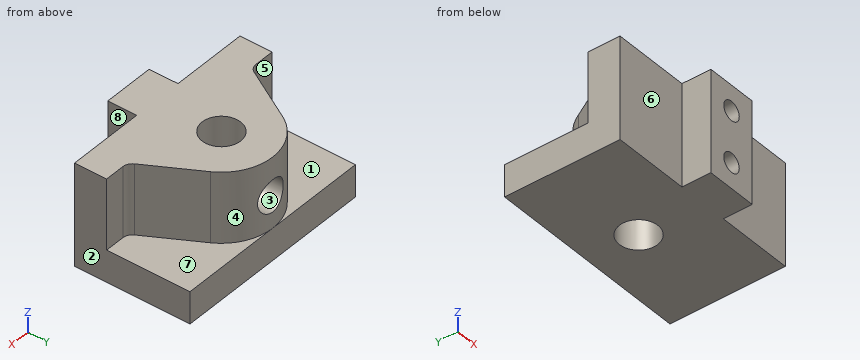
from build123d import *

# Parameters (mm, degrees)
BOSS_EXTRUDE1_DEPTH       = 36
CUT_EXTRUDE6_DEPTH        = 22
SKETCH11_R                = 6.000000000000001
CUT_EXTRUDE7_DEPTH        = 58.827329183593626
SKETCH12_W                = 16
SKETCH12_H                = 32
BOSS_EXTRUDE2_DEPTH       = 9
F_1_0MM_DOWEL_HOLE1_D     = 6
F_1_0MM_DOWEL_HOLE1_DEPTH = 16
F_1_0MM_DOWEL_HOLE1_TIP   = 1.8025818570826808


# Read off the part's stored shape, not the designer's step: CBORE for M6 Hex Socket Head Cap Screw2
with BuildPart() as part:
    # Sketch1 → Boss-Extrude1 (new body)
    with BuildSketch(Plane(origin=(0, 0, 0), x_dir=(1, 0, 0), z_dir=(0, 1, 0))):
        Polygon((-32.000000000000014, 16), (32, 16), (32, -16), (-32.00000000000001, -16), align=None)
    extrude(amount=BOSS_EXTRUDE1_DEPTH)

    # Sketch2 → Cut-Extrude6 (cut)
    with BuildSketch(Plane.XY.offset(16)):
        with BuildLine():
            Line((0.00047501965244123, 36), (-32.00000000000001, 36))
            Line((-32.00000000000001, 36), (-32.00000000000001, 10))
            Line((-32.00000000000001, 10), (-25.751640415984067, 10))
            ThreePointArc((-25.751640415984067, 10), (-24.238970505556754, 10.409280072626942), (-23.139037695662964, 11.5254468386081))
            Line((-23.139037695662964, 11.5254468386081), (-14.249494850462119, 27.275875122834456))
            ThreePointArc((-14.249494850462119, 27.275875122834453), (-8.35374541517065, 33.645768615897694), (0.00047501965243812, 36.00000000705136))
        make_face()
        with BuildLine():
            Line((31.999999999999993, 36), (0.00047501965244123, 36))
            ThreePointArc((0.00047501965243812, 36.00000000705136), (8.07302482579058, 33.814265808302636), (13.940018609128462, 27.85424246049306))
            Line((13.940018609128462, 27.85424246049306), (23.139425445581196, 11.527329539979691))
            ThreePointArc((23.139425445581196, 11.527329539979691), (24.239486779956046, 10.409825162265975), (25.753089868605628, 10))
            Line((25.753089868605628, 10), (32, 10.000000000000002))
            Line((32, 10.000000000000002), (32, 36))
        make_face()
    extrude(amount=-CUT_EXTRUDE6_DEPTH, mode=Mode.SUBTRACT)

    # Sketch11 → Cut-Extrude7 (cut, through all)
    with BuildSketch(Plane.XY.offset(16)):
        with Locations((0.00047501966492051, 20.000000007051366)):
            Circle(SKETCH11_R)
    extrude(amount=-CUT_EXTRUDE7_DEPTH, mode=Mode.SUBTRACT)

    # Sketch12 → Boss-Extrude2 (add)
    with BuildSketch(Plane.XZ):
        Rectangle(SKETCH12_W, SKETCH12_H)
    extrude(amount=BOSS_EXTRUDE2_DEPTH)

    # CBORE for M6 Hex Socket Head Cap Scr 2 → CBORE for M6 Hex Socket Head Cap Screw2 (revolve, cut)
    with BuildSketch(Plane(origin=(0.121141314, 0.00073091, 3.999999998), x_dir=(0.9999817987234716, 0.006033425376210058, 0), z_dir=(0, 0, -1))):
        Polygon((3, -29.599633116), (3, -25.195487191), (0, -25.195487191), (0, -35.999736435), (5, -35.999736435), (5, -29.599633116), align=None)
    revolve(axis=Axis((0.121141314, 0.00073091, 3.999999998), (0.006033425376210058, -0.9999817987234716, 0)), mode=Mode.SUBTRACT)

    # Ø1.0mm Dowel Hole1
    with Locations(Plane(origin=(0, -9, 0), x_dir=(-1, 0, 0), z_dir=(0, -1, 0))):
        with Locations((0, 8), (0, -8)):
            Hole(F_1_0MM_DOWEL_HOLE1_D / 2, depth=F_1_0MM_DOWEL_HOLE1_DEPTH)
            with Locations((0, 0, -(F_1_0MM_DOWEL_HOLE1_DEPTH + F_1_0MM_DOWEL_HOLE1_TIP / 2))):  # 118° drill point
                Cone(0, F_1_0MM_DOWEL_HOLE1_D / 2, F_1_0MM_DOWEL_HOLE1_TIP, mode=Mode.SUBTRACT)


solid = part.part
CAD build for the part. Positions are in the model's coordinates, mm. Face numbers are marked on the shaded views. A direction names the side the tool comes from. Coordinates: 2 decimals unless noted, no trailing zeros. Write each loop counter-clockwise with the first axis right and the second up, starting at its lowest first coordinate (ties: lowest second). Pieces come first, ordered by that corner, then holes. Notation, with made-up numbers: (42, -16.75) - (72, -16.75) arc R21 ccw to (72, -10.75) - close; hole circle Ø9 at (63, 66.25). An arc over 180 degrees is marked (long way). Use a Markdown table: item, result. Add a question column.
Item 1: Band-saw the part on D-D, the plane z = 2.5. Give the cut face in (x, y), and give its area (3 significant figures).
Item 2: Flat gauge pins, fed straight in: pin 1 (3 mm diameter, centred on y = 21.5, z = 9, fed in from -X); pin 2 (12 mm diameter, centred on y = 21, z = 7.5, fed in from +X); pin 3 (2.5 mm diameter, centred on y = -3.5, z = -7.5, fed in from +X). Where does each tip first touch, or does it go through?
Item 3: Drill centre lines: L1, parallel to Z at x = 0, y = 3.25; L2, parallel to Y at x = 26.5, z = -10; L3, parallel to Z at x = -29, y = 21. Where is each one in solid material? Low to high. Write a range as from..to.
Item 4: Band-saw the part on B-B, the plane y = 20. Give the cut face in (x, z).
Item 5: Band-saw the part on A-A, the plane z = -3. Give the cut face in (x, y).
Item 6: 3-axis set-ups, long thin cutter, end or side, ignore diameter. For the marked faces 4, 5, 6, 7 and 8: which of +Z, -Z, +X, -X, +Y, -Y reach the whole face in a straight line?
Item 7: Mould opens along X. For the marked faces 1, 2 and 3 say: pulls with the +X half, pulls with the -X half, needs draft (parallel to the pull), parting line crosses it, or undercut.
Item 8: Band-saw the part on C-C, the plane x = -27. Give the cut face in (y, z).
Numbers:
| question | item | result |
|---|---|---|
| 1 | outline | (-32, 0) - (-8, 0) - (-8, -9) - (8, -9) - (8, 0) - (32, 0) - (32, 10) - (25.75, 10) arc R3 cw to (23.14, 11.53) - (13.94, 27.85) arc R16 ccw to (4.68, 35.3) - (4.71, 29.63) - (2.54, 29.62) - (2.57, 25.42) arc R6 cw (long way) to (-2.63, 25.39) - (-2.66, 29.58) - (-4.83, 29.57) - (-4.86, 35.24) arc R16 ccw to (-14.25, 27.28) - (-23.14, 11.53) arc R3 cw to (-25.75, 10) - (-32, 10) - close |
| 1 | area | 1,430 mm2 |
| 2 | pin 1 | x = -18.36 |
| 2 | pin 2 | x = 21.18 |
| 2 | pin 3 | x = 8 |
| 3 | L1 | -16..-11, -5..5, 11..16 |
| 3 | L2 | 0..36 |
| 3 | L3 | -16..-6 |
| 4 | outline | (-32, -16) - (-6, -16) - (-6, 16) - (-18.36, 16) - (-18.36, -6) - (-32, -6) - close; (6, -16) - (32, -16) - (32, -6) - (18.37, -6) - (18.37, 16) - (6, 16) - close |
| 5 | outline | (-32, 0) - (-8, 0) - (-8, -9) - (8, -9) - (8, 0) - (32, 0) - (32, 10) - (25.75, 10) arc R3 cw to (23.14, 11.53) - (13.94, 27.85) arc R16 ccw to (-14.25, 27.28) - (-23.14, 11.53) arc R3 cw to (-25.75, 10) - (-32, 10) - close; hole circle Ø12 at (0, 20) |
| 6 | face 4 | +Z, +Y |
| 6 | face 5 | +Z, -X, +Y |
| 6 | face 6 | +Z, -Z, -X, -Y |
| 6 | face 7 | +Z, +X, +Y |
| 6 | face 8 | +Z, -Z, +X, -Y |
| 7 | face 1 | needs draft |
| 7 | face 2 | pulls with the +X half |
| 7 | face 3 | undercut |
| 8 | outline | (0, -16) - (36, -16) - (36, -6) - (10, -6) - (10, 16) - (0, 16) - close |
